Study the drawing (mm; zero at the part's minimum x, y, z) and answer. A direction names the side the tool comes from. Coordinates: 2 decimals unless noted, no trailing zeros. Order: outer loops, then holes, each group sorted by start corner. A loop starts at its lowest first (then second) coordinate and runs counter-clockwise, first axis right, second up. Notation, with made-up numbers: (59.5, 62.5) -> (96.5, 62.5) arc R20 cw to (96.5, 86.5) -> close; hole circle Ø6 at (-13, 54). An arc over 180 degrees is marked (long way). One line per question, with ' | ' between items.
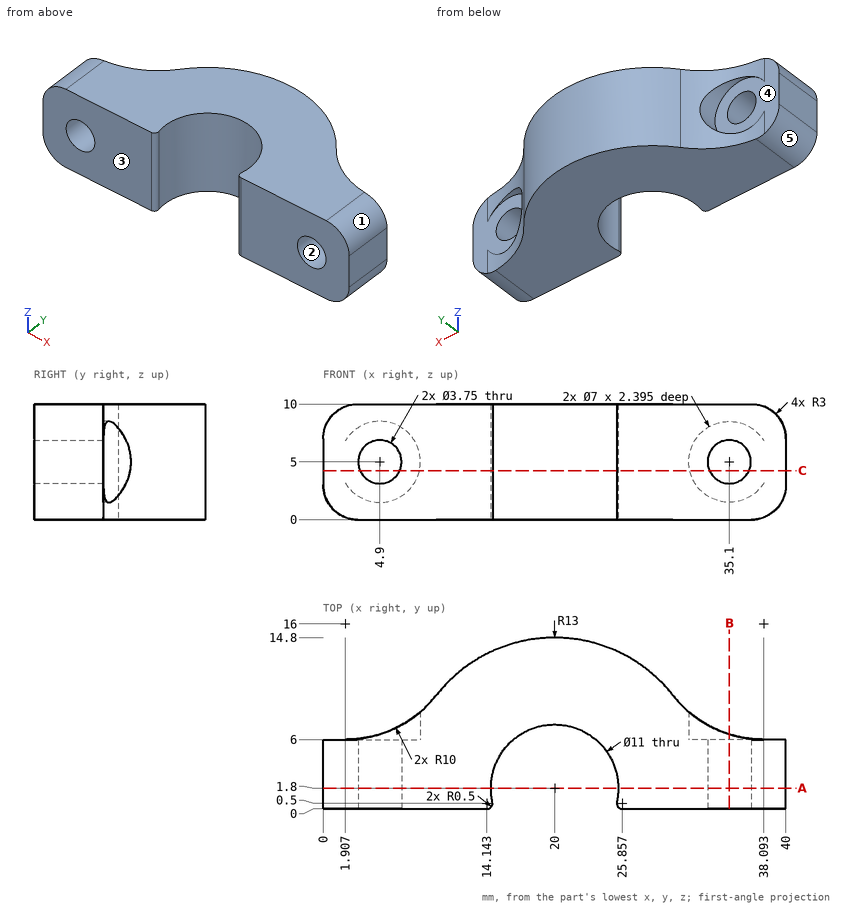
Item 1: Section C-C, the plane z = 4.25 is taken. Give the vertices of the cut face in (x, y).
Computed values:
outline: (0, 0) -> (3.18, 0) -> (3.18, 6) -> (0, 6) -> close; (6.62, 0) -> (14.14, 0) arc R0.5 ccw to (14.63, 0.61) arc R5.5 cw (long way) to (25.37, 0.61) arc R0.5 ccw to (25.86, 0) -> (33.38, 0) -> (33.38, 6) -> (31.68, 6) -> (31.68, 8.33) arc R10 cw to (30.23, 9.83) arc R13 ccw to (9.77, 9.83) arc R10 cw to (8.32, 8.33) -> (8.32, 6) -> (6.62, 6) -> close; (36.82, 0) -> (40, 0) -> (40, 6) -> (36.82, 6) -> close
Item 2: Each of these flat-tipped pins is pushed along its axis until it touches: pin 1 Ø6 at (y, z) = (7, 4) entering from +X; pin 2 Ø4 at (x, z) = (4.9, 5) entering from +Y; pin 3 Ø2 at (x, z) = (4.9, 5) entering from +Y; pin 4 Ø1 at (y, z) = (10, 8) entering from +X (1 decimal). Where does it stop, or does it pass through?
Computed values:
pin 1: stops at x = 40 | pin 2: stops at y = 6 | pin 3: passes through | pin 4: stops at x = 30.5
Item 3: For the marked faces 4 and 5, determine the directions among +Z, -Z, +X, -X, +Y, -Y from which every point of the face is accessible in a straight line to the end or side of a thin tool.
Computed values:
face 4: +Y | face 5: -Z, -X, +Y, -Y
Item 4: Determine the mould class of the marked faces 1, 2 and 3 for opening direction Z: pulls with the +Z half, pulls with the -Z half, needs draft (parallel to the pull), parting line crosses it, or undercut.
Computed values:
face 1: pulls with the +Z half | face 2: undercut | face 3: needs draft
Item 5: Section B-B, the plane x = 35.1 is taken. Give the vertices of the cut face in (y, z) (1 decimal).
Computed values:
outline: (0, 0) -> (6.5, 0) -> (6.5, 1.5) -> (6, 1.5) -> (6, 3.1) -> (0, 3.1) -> close; (0, 6.9) -> (6, 6.9) -> (6, 8.5) -> (6.5, 8.5) -> (6.5, 10) -> (0, 10) -> close
Item 6: Find the intervals of material crossed by L1, parallel to X at y = 3.5, z = 5 (1 decimal); L2, parallel to Z at x = 35, y = 5; L3, parallel to Y at x = 37.5, z = 5.5, in increasing order.
Computed values:
L1: x = 0 to 3, 6.8 to 14.8, 25.2 to 33.2, 37 to 40 | L2: z = 0 to 3.13, 6.87 to 10 | L3: y = 0 to 6
Item 7: Section A-A, the plane y = 1.8 is taken. Count the separate pieces of the cut face and the enclosed holes in it, plus the area to 3 significant figures.
Computed values:
separate pieces: 2 | enclosed holes: 2 | area: 260 mm^2
